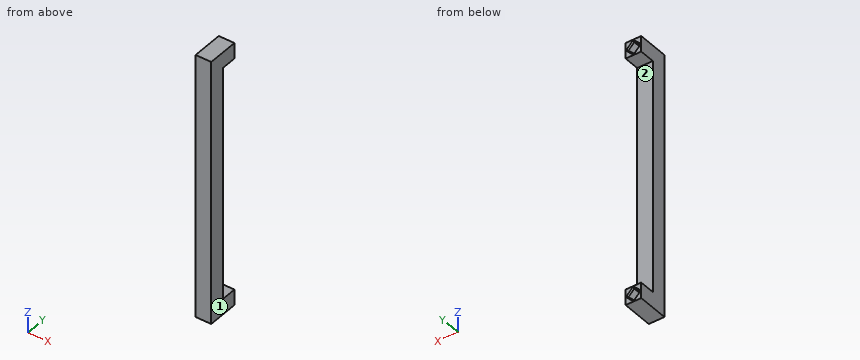
from build123d import *

# Parameters (mm, degrees)
BOSS_EXTRUDE1_DEPTH = 8.466666667
CUT_EXTRUDE1_DEPTH  = 5.08
CHAMFER1_SIZE       = 0.635


with BuildPart() as part:
    # Sketch1 → Boss-Extrude1 (new body)
    with BuildSketch(Plane(origin=(0, 0, 0), x_dir=(0, 0, -1), z_dir=(1, 0, 0))):
        Polygon((-71.466673, 8.466666667), (-71.466673, -8.466666667), (71.466673, -8.466666667), (71.466673, 8.466666667), (63.000006333, 8.466666667), (63.000006333, 0), (-63.000006333, 0), (-63.000006333, 8.466666667), align=None)
    extrude(amount=BOSS_EXTRUDE1_DEPTH)

    # Sketch2 → Cut-Extrude1 (cut)
    with BuildSketch(Plane(origin=(0, 8.466666667, 0), x_dir=(1, 0, 0), z_dir=(0, 1, 0))):
        Polygon((1.058333333, -67.233339667), (4.233333333, -64.058339667), (7.408333333, -67.233339667), (4.233333333, -70.408339667), align=None)
        Polygon((1.058333333, 67.233339667), (4.233333333, 70.408339667), (7.408333333, 67.233339667), (4.233333333, 64.058339667), align=None)
    extrude(amount=-CUT_EXTRUDE1_DEPTH, mode=Mode.SUBTRACT)

    # Chamfer1
    chamfer1_edges = [part.edges().sort_by_distance(p)[0] for p in [
        (2.645833333, 3.386666667, 68.820839667),
        (2.645833333, 3.386666667, 65.645839667),
        (5.820833333, 3.386666667, 65.645839667),
        (5.820833333, 3.386666667, 68.820839667),
        (2.645833333, 8.466666667, 68.820839667),
        (5.820833333, 8.466666667, 68.820839667),
        (5.820833333, 8.466666667, 65.645839667),
        (2.645833333, 8.466666667, 65.645839667),
        (2.645833333, 3.386666667, -65.645839667),
        (2.645833333, 3.386666667, -68.820839667),
        (5.820833333, 3.386666667, -68.820839667),
        (5.820833333, 3.386666667, -65.645839667),
        (2.645833333, 8.466666667, -65.645839667),
        (5.820833333, 8.466666667, -65.645839667),
        (5.820833333, 8.466666667, -68.820839667),
        (2.645833333, 8.466666667, -68.820839667),
    ]]
    chamfer(chamfer1_edges, length=CHAMFER1_SIZE)


solid = part.part
Work out the finished part from the listing and answer in its coordinate system (mm). Face numbers are marked on the shaded views. Round coordinates to 2 decimals unless told otherwise and drop trailing zeros. Write each loop counter-clockwise with the first axis right and the second up, starting at its lowest first coordinate (ties: lowest second). Pieces come first, ordered by that corner, then holes.
1) Straight lines are drawn through the part: line 1 (Z direction, x = 7.25, y = 3.5); line 2 (Y direction, x = 2.75, z = 43). For each, find the intervals that lie inside material, in ascending order.
2) A cutting plane is placed at B-B (z = -38). Give the vertices of the cut face in (x, y), plus the area to 3 significant figures.
3) A cutting plane is placed at A-A (y = 6.25). Give the vertices of the cut face in (x, z), plus the area to 3 significant figures.
4) The mould has two halves that part along Z. Classify the marked faces 1 and 2: pulls with the +Z half, pulls with the -Z half, needs draft (parallel to the pull), parting line crosses it, or undercut.
Completed:
1. line 1: z = -71.47 to -63, 63 to 71.47
1. line 2: y = -8.47 to 0
2. outline: (0, -8.47) - (8.47, -8.47) - (8.47, 0) - (0, 0) - close
2. area: 71.7 mm2
3. outline: (0, -71.47) - (8.47, -71.47) - (8.47, -63) - (0, -63) - close; (0, 63) - (8.47, 63) - (8.47, 71.47) - (0, 71.47) - close; hole (1.06, -67.23) - (4.23, -70.41) - (7.41, -67.23) - (4.23, -64.06) - close; hole (1.06, 67.23) - (4.23, 64.06) - (7.41, 67.23) - (4.23, 70.41) - close
3. area: 103 mm2
4. face 1: needs draft
4. face 2: undercut
